Source: three-view drawing plus pictorial views. Frame: mm from the lowest corner of the part. A direction names the side the tool comes from. Coordinates: 2 decimals unless noted, no trailing zeros. Loops run counter-clockwise (first coordinate to the right, second up) from the corner with the lowest first, then second, coordinate; pieces in that order, holes last.
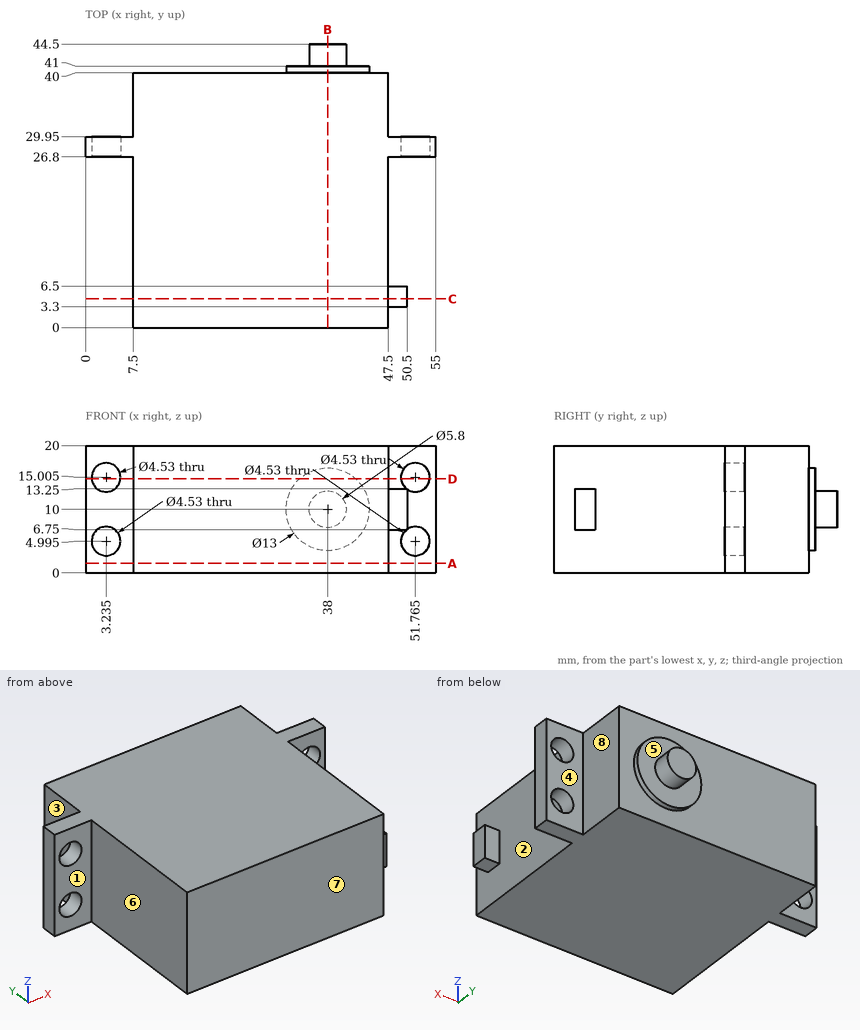
Q1. Section query D-D on z = 14.75. Return the cut outline in (x, y).
Q2. First-contact query: pin 1 Ø3 at (y, z) = (35.5, 6.5) entering from +X; pin 2 Ø3.5 at (x, z) = (51.765, 4.995) entering from +Y; pin 3 Ø0.9 at (x, y) = (48.5, 5) entering from -Z; pin 4 Ø6 at (x, z) = (52, 13) entering from -Y. Flat tips, straight axial feed; report the tip coordinate or a pass-through.
Q3. Material intervals for line 1 along X through (y, z) = (29, 15); line 2 along Y through (x, z) = (34.5, 17.5); line 3 along X through (y, z) = (2, 1.75), sorted ascending.
Q4. Draft query along Y for the marked faces 1, 2, 3 and 4. Return one class per face: released by +Y, released by -Y, zero draft, split by the parting line, or undercut.
Q5. Section query A-A on z = 1.5. Return the cut outline in (x, y).
Q6. Reachability of the marked faces 5, 6, 7 and 8 from +Z, -Z, +X, -X, +Y, -Y: full face, straight path, thin tool, end or side. Return the list, or none.
Q7. Section query C-C on y = 4.5. Return the cut outline in (x, z).
Q8. Section query B-B on x = 38. Return the cut outline in (y, z).
Resolved:
1. outline: (0, 26.8) - (0.98, 26.8) - (0.98, 29.95) - (0, 29.95) - close; (5.49, 26.8) - (7.5, 26.8) - (7.5, 0) - (47.5, 0) - (47.5, 26.8) - (49.51, 26.8) - (49.51, 29.95) - (47.5, 29.95) - (47.5, 40) - (42.44, 40) - (42.44, 41) - (33.56, 41) - (33.56, 40) - (7.5, 40) - (7.5, 29.95) - (5.49, 29.95) - close; (54.02, 26.8) - (55, 26.8) - (55, 29.95) - (54.02, 29.95) - close
2. pin 1: stops at x = 47.5
2. pin 2: passes through
2. pin 3: stops at z = 6.75
2. pin 4: stops at y = 3.3
3. line 1: x = 0 to 0.97, 5.5 to 49.5, 54.03 to 55
3. line 2: y = 0 to 40
3. line 3: x = 7.5 to 47.5
4. face 1: released by -Y
4. face 2: undercut
4. face 3: zero draft
4. face 4: released by +Y
5. outline: (0, 26.8) - (7.5, 26.8) - (7.5, 0) - (47.5, 0) - (47.5, 26.8) - (55, 26.8) - (55, 29.95) - (47.5, 29.95) - (47.5, 40) - (7.5, 40) - (7.5, 29.95) - (0, 29.95) - close
6. face 5: +Y
6. face 6: +Z, -Z, -X, -Y
6. face 7: +Z, -Z, +X, -X, -Y
6. face 8: +Z, -Z, +X, +Y
7. outline: (7.5, 0) - (47.5, 0) - (47.5, 6.75) - (50.5, 6.75) - (50.5, 13.25) - (47.5, 13.25) - (47.5, 20) - (7.5, 20) - close
8. outline: (0, 0) - (40, 0) - (40, 3.5) - (41, 3.5) - (41, 7.1) - (44.5, 7.1) - (44.5, 12.9) - (41, 12.9) - (41, 16.5) - (40, 16.5) - (40, 20) - (0, 20) - close
